Here's how the part is built. I have some questions about the finished solid (model axes, mm). A direction names the side the tool comes from. Coordinates: 2 decimals unless noted, no trailing zeros. Loops run counter-clockwise (first coordinate to the right, second up) from the corner with the lowest first, then second, coordinate; pieces in that order, holes last. Notation, with made-up numbers: (81.5, 67) - (131.5, 67) arc R33 ccw to (131.5, 105) - close; hole circle Ø6 at (22.25, -2). An arc over 180 degrees is marked (long way). Use a Markdown table: item, result.
```python
from build123d import *

# Parameters (mm, degrees)
BOSS_EXTRUDE1_DEPTH = 279.4
SKETCH3_R           = 2.54
CUT_EXTRUDE1_DEPTH  = 279.4
SKETCH4_R           = 2.54
CUT_EXTRUDE2_DEPTH  = 279.4


with BuildPart() as part:
    # Sketch2 → Boss-Extrude1 (new body)
    with BuildSketch(Plane.XY):
        with BuildLine():
            Line((76.923497933, 16.815560225), (87.550840879, 16.815560225))
            Line((87.550840879, 16.815560225), (87.550840879, 14.275560225))
            Line((87.550840879, 14.275560225), (74.850840879, 14.275560225))
            ThreePointArc((74.850840879, 14.275560225), (53.771488035, 53.99136111), (13.97, 74.908471484))
            Line((13.97, 74.908471484), (13.97, 87.608471484))
            Line((13.97, 87.608471484), (16.51, 87.608471484))
            Line((16.51, 87.608471484), (16.51, 76.989658396))
            ThreePointArc((16.51, 76.989658396), (55.566943021, 55.788013437), (76.923497933, 16.815560225))
        make_face()
    extrude(amount=BOSS_EXTRUDE1_DEPTH)

    # Sketch3 → Cut-Extrude1 (cut)
    with BuildSketch(Plane(origin=(16.51, 0, 0), x_dir=(0, 0, -1), z_dir=(1, 0, 0))):
        with Locations((-12.7, 82.528471484)):
            Circle(SKETCH3_R)
        with Locations((-60.96, 82.528471484)):
            Circle(SKETCH3_R)
        with Locations((-109.22, 82.528471484)):
            Circle(SKETCH3_R)
        with Locations((-157.48, 82.528471484)):
            Circle(SKETCH3_R)
        with Locations((-205.74, 82.528471484)):
            Circle(SKETCH3_R)
        with Locations((-254, 82.528471484)):
            Circle(SKETCH3_R)
    extrude(amount=-CUT_EXTRUDE1_DEPTH, mode=Mode.SUBTRACT)

    # Sketch4 → Cut-Extrude2 (cut)
    with BuildSketch(Plane.XZ.offset(-14.275560225)):
        with Locations((82.470840879, 12.7)):
            Circle(SKETCH4_R)
        with Locations((82.470840879, 60.96)):
            Circle(SKETCH4_R)
        with Locations((82.470840879, 109.22)):
            Circle(SKETCH4_R)
        with Locations((82.470840879, 157.48)):
            Circle(SKETCH4_R)
        with Locations((82.470840879, 205.74)):
            Circle(SKETCH4_R)
        with Locations((82.470840879, 254)):
            Circle(SKETCH4_R)
    extrude(amount=-CUT_EXTRUDE2_DEPTH, mode=Mode.SUBTRACT)


solid = part.part
```
Q1. If we mould it in two halves opening along Y, with no side actions, what happens to faces 1 (the face through (55.12, 56.23, 137.74)), 2 (the face through (15.258, 82.64, 208.278)), 3 (the face through (81.92, 15.53, 251.52)), 4 (the face through (81, 14.276, 138))? For each: pulls with the +Y half, pulls with the -Y half, needs draft (parallel to the pull), parting line crosses it, or undercut.
Check values:
| item | result |
|---|---|
| face 1 | pulls with the +Y half |
| face 2 | undercut |
| face 3 | needs draft |
| face 4 | pulls with the -Y half |
Q2. I want a section at C-C, the plane y = 72. Write out the boundary of the cut face in (x, z), then the cut area to 3 significant figures.
Check values:
| item | result |
|---|---|
| outline | (24.95, 0) - (31.87, 0) - (31.87, 279.4) - (24.95, 279.4) - close |
| area | 1,940 mm^2 |
Q3. I want a section at B-B, the plane z = 53. Write out the boundary of the cut face in (x, y), then the cut area to 3 significant figures.
Check values:
| item | result |
|---|---|
| outline | (13.97, 74.91) arc R76.2 cw to (74.85, 14.28) - (87.55, 14.28) - (87.55, 16.82) - (76.92, 16.82) arc R78.74 ccw to (16.51, 76.99) - (16.51, 87.61) - (13.97, 87.61) - close |
| area | 290 mm^2 |
Q4. I want a section at D-D, the plane x = 52.5. Write out the boundary of the cut face in (y, z).
Check values:
| item | result |
|---|---|
| outline | (55.23, 0) - (58.68, 0) - (58.68, 279.4) - (55.23, 279.4) - close |
Q5. I want a section at A-A, the plane z = 254. Write out the boundary of the cut face in (x, y), then the cut area to 3 significant figures.
Check values:
| item | result |
|---|---|
| outline | (13.97, 74.91) arc R76.2 cw to (74.85, 14.28) - (79.93, 14.28) - (79.93, 16.82) - (76.92, 16.82) arc R78.74 ccw to (16.51, 76.99) - (16.51, 79.99) - (13.97, 79.99) - close; (13.97, 85.07) - (16.51, 85.07) - (16.51, 87.61) - (13.97, 87.61) - close; (85.01, 14.28) - (87.55, 14.28) - (87.55, 16.82) - (85.01, 16.82) - close |
| area | 264 mm^2 |
Q6. Which directions (+Z, -Z, +X, -X, +Y, -Y) give clear straight access to the entire face, cutting with the end or side of a thin tool? Please do faces 5 (the face through (16.51, 82, 138)), 6 (the face through (15.26, 81.56, 106.87)).
Check values:
| item | result |
|---|---|
| face 5 | +Z, -Z, +X, +Y |
| face 6 | +X, -X |
Q7. Please list where these lines run through material, in increasing order: L1, parallel to X at y = 78, z = 121; L2, parallel to Y at x = 78, z = 150.5; L3, parallel to Y at x = 42, z = 265. Write a range as from..to.
Check values:
| item | result |
|---|---|
| L1 | 13.97..16.51 |
| L2 | 14.28..16.82 |
| L3 | 63.58..66.6 |
Q8. Will these pins go through, and if not, where does the flat tip stop? P1, Ø8, axis at y = 65.5, z = 234.5, coming from the -X side; P2, Ø6.5, axis at x = 82.47, z = 254, coming from the -Y side; P3, Ø8, axis at x = 82.47, z = 60.96, coming from the +Y side; P4, Ø12, axis at y = 64.5, z = 110.5, coming from the +X side.
Check values:
| item | result |
|---|---|
| P1 | x = 31.24 |
| P2 | y = 14.28 |
| P3 | y = 16.82 |
| P4 | x = 52.7 |
